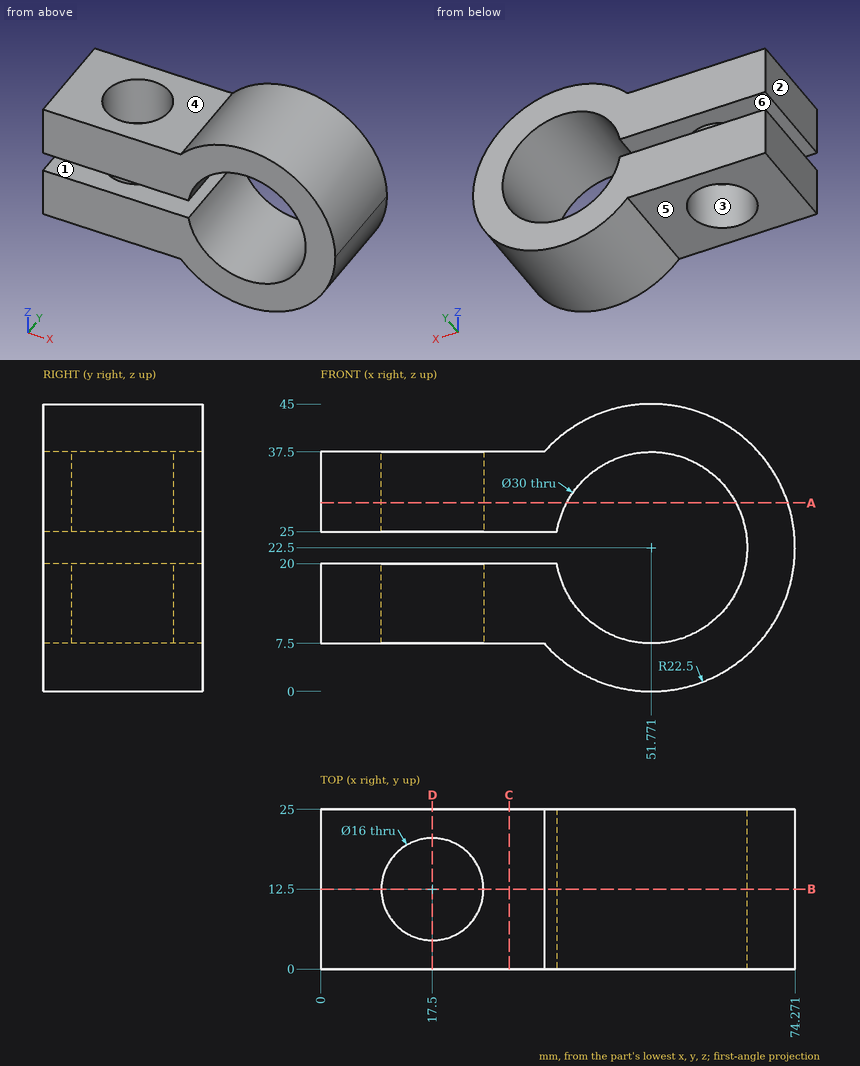
Source: three-view drawing plus pictorial views. Frame: mm from the lowest corner of the part. A direction names the side the tool comes from. Give positions to 0.01 mm unless a question says otherwise; leave off trailing zeros. Order: outer loops, then holes, each group sorted by start corner. A loop starts at its lowest first (then second) coordinate and runs counter-clockwise, first axis right, second up.
1. Section A-A on z = 29.5. Return the cut outline in (x, y) (1 decimal).
Derived:
outline: (0, 0) - (38.5, 0) - (38.5, 25) - (0, 25) - close; (65, 0) - (73.2, 0) - (73.2, 25) - (65, 25) - close; hole circle Ø16 at (17.5, 12.5)
2. Mould query, pull axis X, two halves, no side actions, for the marked faces 1, 2 and 3. Classes: released by +X, released by -X, zero draft, split by the parting line, or undercut.
Derived:
face 1: zero draft
face 2: released by -X
face 3: undercut
3. Reachability of the marked faces 4, 5 and 6 from +Z, -Z, +X, -X, +Y, -Y: full face, straight path, thin tool, end or side. Return the list, or none.
Derived:
face 4: +Z, -X, +Y, -Y
face 5: -Z, -X, +Y, -Y
face 6: -X, +Y, -Y
4. Section B-B on y = 12.5. Return the cut outline in (x, z).
Derived:
outline: (0, 7.5) - (9.5, 7.5) - (9.5, 20) - (0, 20) - close; (0, 25) - (9.5, 25) - (9.5, 37.5) - (0, 37.5) - close; (25.5, 7.5) - (35, 7.5) arc R22.5 ccw (long way) to (35, 37.5) - (25.5, 37.5) - (25.5, 25) - (36.98, 25) arc R15 cw (long way) to (36.98, 20) - (25.5, 20) - close
5. Material intervals for L1, parallel to Z at x = 10.5, y = 1.25; L2, parallel to Y at x = 17.5, z = 11.5; L3, parallel to X at y = 6.75, z = 18 (1 decimal), sorted ascending.
Derived:
L1: z = 7.5 to 20, 25 to 37.5
L2: y = 0 to 4.5, 20.5 to 25
L3: x = 0 to 11.9, 23.1 to 37.5, 66.1 to 73.8
6. Section C-C on x = 29.5. Return the cut outline in (y, z), and give its area (3 significant figures).
Derived:
outline: (0, 7.5) - (25, 7.5) - (25, 20) - (0, 20) - close; (0, 25) - (25, 25) - (25, 37.5) - (0, 37.5) - close
area: 625 mm2
7. Pin query (flat end, axial travel): pin 1 (1 mm diameter, centred on x = 9, y = 4.5, fed in from +Z); pin 2 (12 mm diameter, centred on y = 9, z = 36, fed in from +X); pin 3 (13 mm diameter, centred on x = 17.5, y = 12.5, fed in from +Z); pin 4 (6 mm diameter, centred on y = 15, z = 11.5, fed in from +X). Return the tip coordinate at first contact, or that it passes through.
Derived:
pin 1: stops at z = 37.5
pin 2: stops at x = 72.98
pin 3: passes through
pin 4: stops at x = 72.8
8. Section D-D on x = 17.5. Return the cut outline in (y, z).
Derived:
outline: (0, 7.5) - (4.5, 7.5) - (4.5, 20) - (0, 20) - close; (0, 25) - (4.5, 25) - (4.5, 37.5) - (0, 37.5) - close; (20.5, 7.5) - (25, 7.5) - (25, 20) - (20.5, 20) - close; (20.5, 25) - (25, 25) - (25, 37.5) - (20.5, 37.5) - close
